Work out the finished part from the listing and answer in its coordinate system (mm). A direction names the side the tool comes from. Give positions to 0.01 mm unless a question says otherwise; leave off trailing zeros. Order: outer loops, then holes, each group sorted by start corner. A loop starts at its lowest first (then second) coordinate and runs counter-clockwise, first axis right, second up. Notation, with made-up numbers: (-2.5, 46) -> (54.5, 46) arc R21 cw to (54.5, 64) -> close; hole circle Ø5 at (4.25, 29). An arc over 180 degrees is marked (long way). Use a Markdown table: item, result. Add a question column.
```python
from build123d import *

# Parameters (mm, degrees)
SKETCH_1_R               = 68
SKETCH_1_R_2             = 65
EXTRUDE_1_DEPTH          = 55
SKETCH_2_R               = 68
EXTRUDE_1_2_DEPTH        = 4
FILLET_1_R               = 15
EXTRUDE_2_DEPTH          = 30
SKETCH_4_W               = 50
SKETCH_4_H               = 30
EXTRUDE_3_DEPTH          = 15
CUT_EXTRUDE_1_DEPTH      = 40
CUT_EXTRUDE_2_DEPTH      = 10
CUT_EXTRUDE_2_DEPTH_BACK = 20


with BuildPart() as part:
    # 草图1 → Extrude 1 (new body)
    with BuildSketch(Plane.XY):
        Circle(SKETCH_1_R)
        Circle(SKETCH_1_R_2, mode=Mode.SUBTRACT)
    extrude(amount=EXTRUDE_1_DEPTH)

    # 草图2 → Extrude 1 2 (add)
    with BuildSketch(Plane(origin=(0, 0, 0), x_dir=(-1, 0, 0), z_dir=(0, 0, -1))):
        with Locations(Location((0, 0, 0), (0, 0, 180))):
            Circle(SKETCH_2_R)
    extrude(amount=-EXTRUDE_1_2_DEPTH)

    # 圆角1
    fillet_1_edges = [part.edges().sort_by_distance(p)[0] for p in [
        (-65, 0, 4),
    ]]
    fillet(fillet_1_edges, radius=FILLET_1_R)

    # 草图3 → 凸台-拉伸2 (add)
    with BuildSketch(Plane(origin=(0, 0, 0), x_dir=(-1, 0, 0), z_dir=(0, 0, -1))):
        with BuildLine():
            Line((25, -73), (25, -63.237647015))
            ThreePointArc((25, -63.237647015), (12.724779035, -66.798802373), (0, -68))
            ThreePointArc((0, -68), (-12.724779035, -66.798802373), (-25, -63.237647015))
            Line((-25, -63.237647015), (-25, -73))
            Line((-25, -73), (25, -73))
        make_face()
        with BuildLine():
            ThreePointArc((-25, 63.237647015), (-12.724779035, 66.798802373), (0, 68))
            ThreePointArc((0, 68), (12.724779035, 66.798802373), (25, 63.237647015))
            Line((25, 63.237647015), (25, 73))
            Line((25, 73), (-25, 73))
            Line((-25, 73), (-25, 63.237647015))
        make_face()
    extrude(amount=-EXTRUDE_2_DEPTH)

    # 草图4 → 凸台-拉伸3 (add)
    with BuildSketch(Plane.XZ.offset(73)):
        with Locations((0, 15)):
            Rectangle(SKETCH_4_W, SKETCH_4_H)
    extrude(amount=EXTRUDE_3_DEPTH)

    # 草图5 → 切除-拉伸1 (cut)
    with BuildSketch(Plane(origin=(25, 0, 0), x_dir=(0, 0, -1), z_dir=(1, 0, 0))):
        with BuildLine():
            Line((-18.15, -72.335532476), (-18.15, -75.618823508))
            Line((-18.15, -75.618823508), (-11.85, -75.618823508))
            Line((-11.85, -75.618823508), (-11.85, -72.335532476))
            ThreePointArc((-11.85, -72.335532476), (-15, -71.068823508), (-18.15, -72.335532476))
        make_face()
        with BuildLine():
            Line((-11.85, -75.618823508), (-18.15, -75.618823508))
            Line((-18.15, -75.618823508), (-18.15, -78.902114539))
            ThreePointArc((-18.15, -78.902114539), (-15, -80.168823508), (-11.85, -78.902114539))
            Line((-11.85, -78.902114539), (-11.85, -75.618823508))
        make_face()
    extrude(amount=-CUT_EXTRUDE_1_DEPTH, mode=Mode.SUBTRACT)

    # 草图6 → 切除-拉伸2 (cut, two sides: drawn at the far end of the back side and taken through both)
    with BuildSketch(Plane(origin=(0, 0, 18.15), x_dir=(-1, 0, 0), z_dir=(0, 0, -1)).offset(-CUT_EXTRUDE_2_DEPTH_BACK)):
        with BuildLine():
            ThreePointArc((7.768196181, -75.618823508), (4.968196181, -72.818823508), (2.168196181, -75.618823508))
            Line((2.168196181, -75.618823508), (7.768196181, -75.618823508))
        make_face()
        with BuildLine():
            Line((7.768196181, -75.618823508), (2.168196181, -75.618823508))
            ThreePointArc((2.168196181, -75.618823508), (4.968196181, -78.418823508), (7.768196181, -75.618823508))
        make_face()
    extrude(amount=CUT_EXTRUDE_2_DEPTH + CUT_EXTRUDE_2_DEPTH_BACK, mode=Mode.SUBTRACT)


solid = part.part
```
1) Determine the mould class of faces 1 (the cylindrical face through (-5.3, -78.4, 10)), 2 (the flat face through (55, -35, 55)), 3 (the flat face through (0, 73, 15)) for opening direction Y: released by +Y, released by -Y, zero draft, split by the parting line, or undercut.
2) The part is cut by section A-A, the plane x = 0. Determine the outline of the cut face in (y, z), then the cut area to 3 significant figures.
3) The part is cut by section B-B, the plane z = 14. Determine the outline of the cut face in (x, y), then the cut area to 3 significant figures.
4) Straight lines are drawn through the part: line 1 (Y direction, x = 0, z = 45); line 2 (Z direction, x = -1.5, y = -29.5). For each, find the intervals that lie inside material, in ascending order.
5) Flat-ended cylindrical pins translate along their axes: pin 1 (1.5 mm diameter, centred on x = 13, z = 39.5, fed in from +Y); pin 2 (12.5 mm diameter, centred on y = -70, z = 7.5, fed in from -X); pin 3 (2 mm diameter, centred on y = 21.5, z = 36, fed in from -X); pin 4 (3 mm diameter, centred on x = 2, y = 69, fed in from +Z). Find the tip coordinate at first contact, or state that the pin passes through.
6) The part is cut by section C-C, the plane y = 0. Determine the outline of the cut face in (x, z), then the cut area to 3 significant figures.
7) Which of the six approach directions +Z, -Z, +X, -X, +Y, -Y give full straight-line access (tool end or side, diameter ignored) to faces 4 (the flat face through (-25, 68, 15)), 5 (the cylindrical face through (62, 19.52, 36.75)), 6 (the cylindrical face through (5.28, -80.17, 15.05)), 7 (the flat face through (-25, -75, 15))?
8) The part is cut by section D-D, the plane z = 50. Determine the outline of the cut face in (x, y), then the cut area to 3 significant figures.
A:
| question | item | result |
|---|---|---|
| 1 | face 1 | undercut |
| 1 | face 2 | zero draft |
| 1 | face 3 | released by +Y |
| 2 | outline | (-88, 0) -> (73, 0) -> (73, 30) -> (68, 30) -> (68, 55) -> (65, 55) -> (65, 19) arc R15 cw to (50, 4) -> (-50, 4) arc R15 cw to (-65, 19) -> (-65, 55) -> (-68, 55) -> (-68, 30) -> (-88, 30) -> close; hole (-78.9, 11.85) -> (-72.34, 11.85) arc R4.55 ccw to (-72.34, 18.15) -> (-78.9, 18.15) arc R4.55 ccw to start |
| 2 | area | 1,640 mm^2 |
| 3 | outline | (-25, -88) -> (25, -88) -> (25, -80.06) -> (-15, -80.06) -> (-15, -71.18) -> (25, -71.18) -> (25, -63.24) arc R68 ccw to (25, 63.24) -> (25, 73) -> (-25, 73) -> (-25, 63.24) arc R68 ccw to (-25, -63.24) -> close; hole circle Ø128.28 at (0, 0) |
| 3 | area | 2,650 mm^2 |
| 4 | line 1 | -68 to -65, 65 to 68 |
| 4 | line 2 | 0 to 4 |
| 5 | pin 1 | y = 66.89 |
| 5 | pin 2 | x = -25 |
| 5 | pin 3 | x = -64.84 |
| 5 | pin 4 | z = 55 |
| 6 | outline | (-68, 0) -> (68, 0) -> (68, 55) -> (65, 55) -> (65, 19) arc R15 cw to (50, 4) -> (-50, 4) arc R15 cw to (-65, 19) -> (-65, 55) -> (-68, 55) -> close |
| 6 | area | 947 mm^2 |
| 7 | face 4 | +Z, -Z, -X, +Y |
| 7 | face 5 | +Z |
| 7 | face 6 | +X |
| 7 | face 7 | +Z, -Z, -X, -Y |
| 8 | outline | circle Ø136 at (0, 0); hole circle Ø130 at (0, 0) |
| 8 | area | 1,250 mm^2 |
